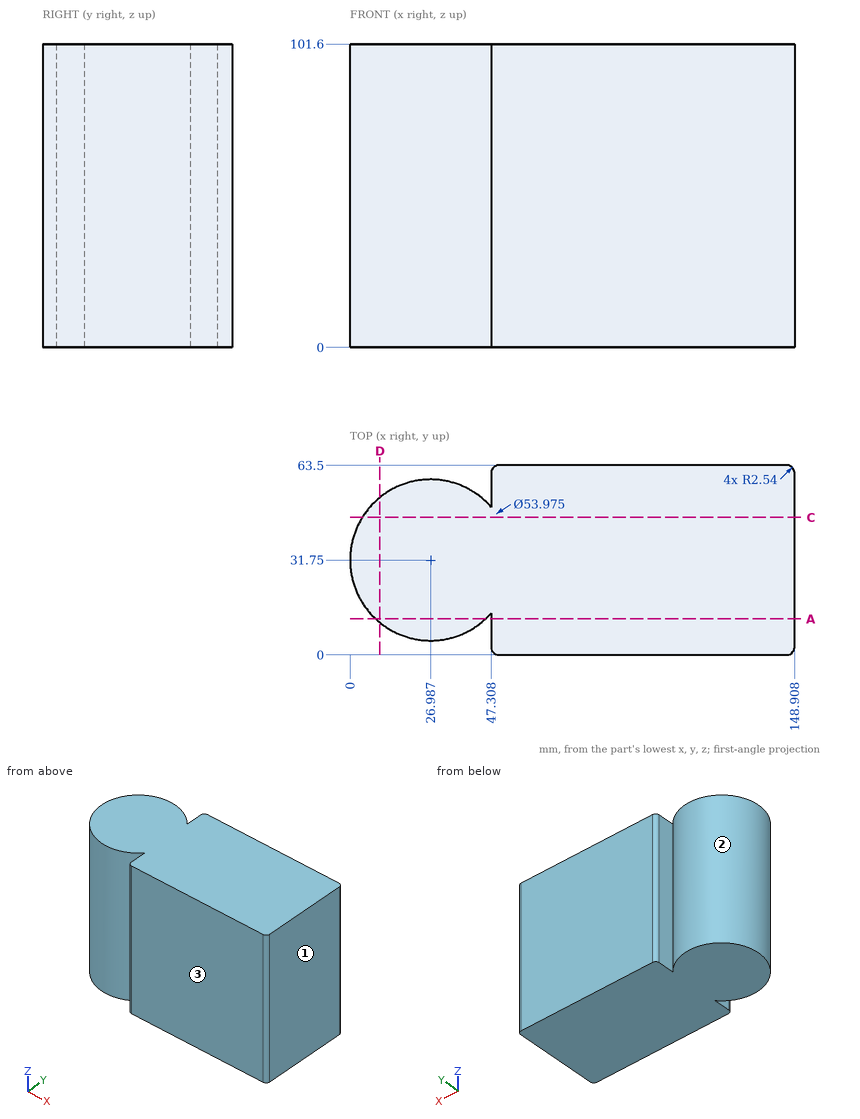
Can you work these out from the drawing? Everything is in mm from the part's minimum corner. Coordinates: 2 decimals unless noted, no trailing zeros. Loops run counter-clockwise (first coordinate to the right, second up) from the corner with the lowest first, then second, coordinate; pieces in that order, holes last.
1) Imagine slicing it at A-A (y = 12). List the corners of the cut face in (x, z) for me (1 decimal), and give its area (3 significant figures).
Reported:
outline: (8.6, 0) - (45.4, 0) - (45.4, 101.6) - (8.6, 101.6) - close; (47.3, 0) - (148.9, 0) - (148.9, 101.6) - (47.3, 101.6) - close
area: 14,100 mm2
2) Thinking about a two-plate mould opening in X: for the marked faces 1, 2 and 3, which applies, released by +X, released by -X, zero draft, split by the parting line, or undercut?
Reported:
face 1: released by +X
face 2: undercut
face 3: zero draft
3) Imagine slicing it at C-C (y = 46). List the corners of the cut face in (x, z) for me.
Reported:
outline: (4.07, 0) - (148.91, 0) - (148.91, 101.6) - (4.07, 101.6) - close
4) Will these pins go through, and if not, where does the flat tip stop? pin 1 Ø12.5 at (y, z) = (55.5, 31) entering from -X; pin 2 Ø9 at (y, z) = (6, 55) entering from -X; pin 3 Ø5 at (x, z) = (38, 20.5) entering from +Y.
Reported:
pin 1: stops at x = 6.44
pin 2: stops at x = 10.35
pin 3: stops at y = 57.36
5) Please list where these lines run through material, in increasing order: line 1 along X through (y, z) = (3, 14.5); line 2 along X through (y, z) = (53.5, 48) (1 decimal); line 3 along X through (y, z) = (56, 92.5) (1 decimal).
Reported:
line 1: x = 47.31 to 148.91
line 2: x = 11 to 43, 47.3 to 148.9
line 3: x = 15.1 to 38.8, 47.3 to 148.9
6) Imagine slicing it at D-D (x = 10). List the corners of the cut face in (y, z) for me, and give its area (3 significant figures).
Reported:
outline: (10.78, 0) - (52.72, 0) - (52.72, 101.6) - (10.78, 101.6) - close
area: 4,260 mm2
